Can you work these out from the drawing? Everything is in mm from the part's minimum corner. A direction names the side the tool comes from. Round coordinates to 2 decimals unless told otherwise and drop trailing zeros. Write each loop counter-clockwise with the first axis right and the second up, starting at its lowest first coordinate (ties: lowest second). Pieces come first, ordered by that corner, then holes. Notation, with made-up numbers: M 29,87 L 79,87 A23 cw 79,118 Z; hole C -17,-38 d11. An arc over 180 degrees is marked long. Use a Markdown table: item, result. Add a question column.
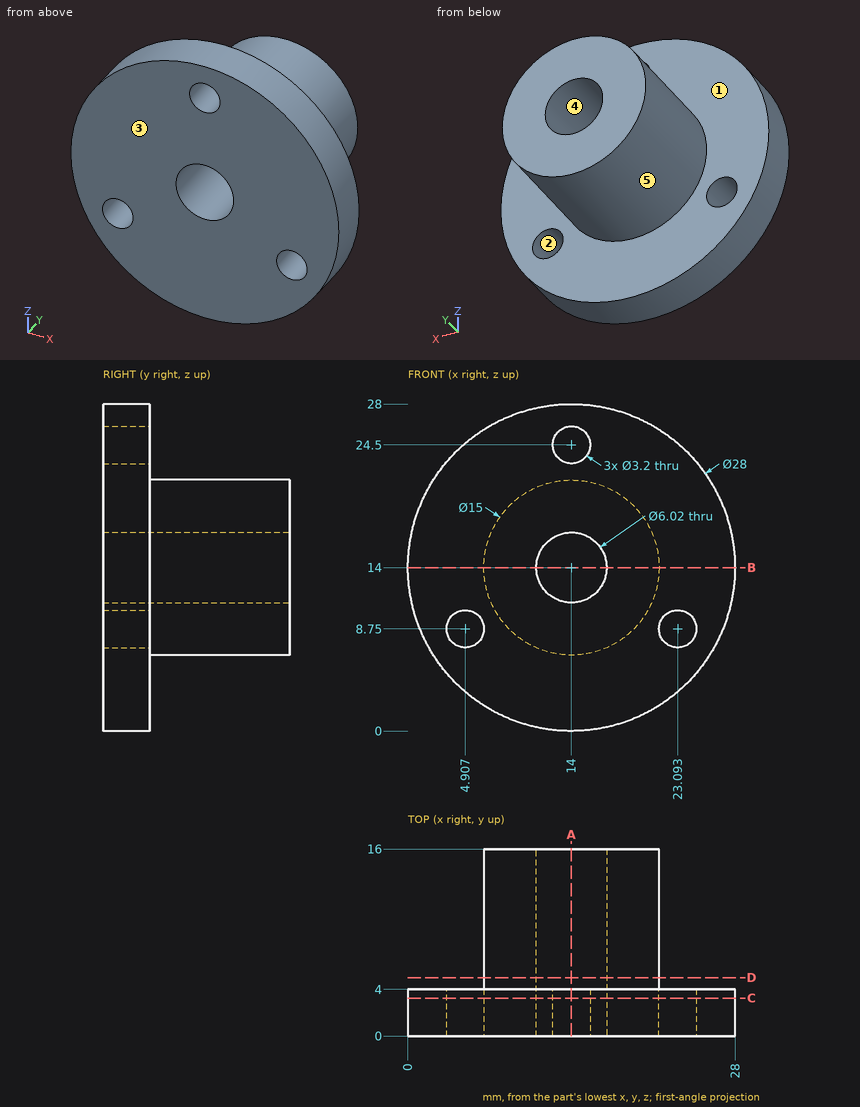
Item 1: For pin 1 Ø4 at (x, y) = (5.5, 7) entering from +Z; pin 2 Ø1.5 at (x, z) = (14.5, 23) entering from -Y; pin 3 Ø1.5 at (x, y) = (8.5, 10) entering from -Z (1 decimal); pin 4 Ø3 at (x, z) = (20.5, 21.5) entering from +Y, each with a flat end and sliding along its axis, tell me the tip position at first contact or that it passes through.
Item 2: I need wall thicknesses on probe 1 along Z at (x, y) = (14, 2.25); probe 2 along X at (y, z) = (2.05, 8.75); probe 3 along Y at (x, z) = (24.25, 11.5). Which ranges of each line are inside material? Lowest first, please. Write a range as from..to.
Item 3: On a 3-axis mill with a long thin cutter (end or side, diameter ignored), from which of +Z, -Z, +X, -X, +Y, -Y can I reach the whole of each face in a straight line? I mean the marked faces 1 and 2. Say none if no direction works.
Item 4: Imagine slicing it at C-C on y = 3.25. List the corners of the cut face in (x, z) for me.
Item 5: Imagine slicing it at A-A on x = 14. List the corners of the cut face in (y, z) for me, plus the area to 3 significant figures.
Item 6: Imagine slicing it at B-B on z = 14. List the corners of the cut face in (x, y) for me.
Item 7: If we mould it in two halves opening along Z, with no side actions, what happens to the marked faces 3, 4 and 5? For each: +Z half, -Z half, draft (parallel to the pull), parting line (faces both ways), or undercut.
Item 8: Imagine slicing it at D-D on y = 5. List the corners of the cut face in (x, z) for me, plus the area to 3 significant figures.
The answers:
| question | item | result |
|---|---|---|
| 1 | pin 1 | z = 17.74 |
| 1 | pin 2 | y = 0 |
| 1 | pin 3 | z = 8.2 |
| 1 | pin 4 | y = 4 |
| 2 | probe 1 | 0..10.99, 17.01..22.9, 26.1..28 |
| 2 | probe 2 | 1.02..3.31, 6.51..21.49, 24.69..26.98 |
| 2 | probe 3 | 0..4 |
| 3 | face 1 | +Y |
| 3 | face 2 | +Y, -Y |
| 4 | outline | C 14,14 d28; hole C 4.91,8.75 d3.2; hole C 14,14 d6.02; hole C 14,24.5 d3.2; hole C 23.09,8.75 d3.2 |
| 5 | outline | M 0,0 L 4,0 L 4,6.5 L 16,6.5 L 16,10.99 L 0,10.99 Z; M 0,17.01 L 16,17.01 L 16,21.5 L 4,21.5 L 4,22.9 L 0,22.9 Z; M 0,26.1 L 4,26.1 L 4,28 L 0,28 Z |
| 5 | area | 183 mm² |
| 6 | outline | M 0,0 L 10.99,0 L 10.99,16 L 6.5,16 L 6.5,4 L 0,4 Z; M 17.01,0 L 28,0 L 28,4 L 21.5,4 L 21.5,16 L 17.01,16 Z |
| 7 | face 3 | draft |
| 7 | face 4 | undercut |
| 7 | face 5 | parting line |
| 8 | outline | C 14,14 d15; hole C 14,14 d6.02 |
| 8 | area | 148 mm² |
